```python
from build123d import *

# Parameters (mm, degrees)
SKETCH_1_W              = 40
SKETCH_1_H              = 40
EXTRUDE_1_DEPTH         = 20
SKETCH_2_R              = 6.58
EXTRUDE_2_DEPTH         = 1.8
SKETCH_3_R              = 2.925
EXTRUDE_3_DEPTH         = 3.8
SKETCH_4_W              = 7
SKETCH_4_H              = 20
EXTRUDE_4_DEPTH         = 2.4
HOLE_WIZARD_4_4_4_4_1_D = 4.4
SKETCH_7_W              = 5.7
SKETCH_7_H              = 4
EXTRUDE_5_DEPTH         = 8.5


with BuildPart() as part:
    # 草图1 → 凸台-拉伸1 (new body)
    with BuildSketch(Plane.XY):
        Rectangle(SKETCH_1_W, SKETCH_1_H)
    extrude(amount=EXTRUDE_1_DEPTH)

    # 草图2 → 凸台-拉伸2 (add)
    with BuildSketch(Plane(origin=(0, 20, 0), x_dir=(1, 0, 0), z_dir=(0, 1, 0))):
        with Locations((-10.3, -10)):
            Circle(SKETCH_2_R)
    extrude(amount=EXTRUDE_2_DEPTH)

    # 草图3 → 凸台-拉伸3 (add)
    with BuildSketch(Plane(origin=(0, 21.8, 0), x_dir=(1, 0, 0), z_dir=(0, 1, 0))):
        with Locations((-10.3, -10)):
            Circle(SKETCH_3_R)
    extrude(amount=EXTRUDE_3_DEPTH)

    # 草图4 → 凸台-拉伸4 (add)
    with BuildSketch(Plane(origin=(0, 12.2, 0), x_dir=(1, 0, 0), z_dir=(0, 1, 0))):
        with Locations((-23.5, -10)):
            Rectangle(SKETCH_4_W, SKETCH_4_H)
        with Locations((23.5, -10)):
            Rectangle(SKETCH_4_W, SKETCH_4_H)
    extrude(amount=-EXTRUDE_4_DEPTH)

    # Ø4.4 (4.4) 直径孔1 (through all)
    with Locations(Plane(origin=(0, 12.2, 0), x_dir=(1, 0, 0), z_dir=(0, 1, 0))):
        with Locations((-24.35, -4.95), (-24.35, -15.05), (24.35, -4.95), (24.35, -14.883974449)):
            Hole(HOLE_WIZARD_4_4_4_4_1_D / 2)

    # 草图7 → 凸台-拉伸5 (add)
    with BuildSketch(Plane.ZY.offset(20)):
        with Locations((10, -13.2)):
            Rectangle(SKETCH_7_W, SKETCH_7_H)
    extrude(amount=EXTRUDE_5_DEPTH)


solid = part.part
```
The listing builds one solid part. Answer for the finished solid, in the listing's coordinates (mm). A direction names the side the tool comes from. Coordinates: 2 decimals unless noted, no trailing zeros. Loops run counter-clockwise (first coordinate to the right, second up) from the corner with the lowest first, then second, coordinate; pieces in that order, holes last. Notation, with made-up numbers: (18, 36.5) -> (69, 36.5) arc R23 cw to (69, 64.5) -> close; hole circle Ø4 at (73.5, 25.5). An arc over 180 degrees is marked (long way). Return JSON: item names as keys, results as strings. Group by question number.
(1) A cutting plane is placed at A-A on x = -24.35. Write down the section's boundary in (y, z), and give its area (3 significant figures).
(2) Determine the mould class of faces 6 (the flat face through (0, 20, 10)), 7 (the cylindrical face through (-12.62, 23.67, 11.78)), 8 (the cylindrical face through (-25.37, 10.98, 17)), 9 (the cylindrical face through (-26.45, 10.98, 4.29)) for opening direction Z: released by +Z, released by -Z, zero draft, split by the parting line, or undercut.
(3) Given pin 1 Ø4 at (y, z) = (17, 7.5) entering from -X; pin 2 Ø2.5 at (y, z) = (15, 14.5) entering from +X; pin 3 Ø1.7 at (x, z) = (-22.5, 9) entering from -Y; pin 4 Ø2.5 at (x, z) = (24.35, 14.88) entering from +Y, each flat-ended and moving along its own axis, determine where each tip first touches the part or whether it passes through.
(4) A cutting plane is placed at B-B on z = 6.25. Write down the section's boundary in (x, y), and give its area (3 significant figures).
(5) Which of the six approach directions +Z, -Z, +X, -X, +Y, -Y give full straight-line access (tool end or side, diameter ignored) to faces 1 (the flat face through (-9, 21.8, 13)), 2 (the flat face through (-24, -11.2, 10)), 3 (the flat face through (-27, 11, 10)), 4 (the flat face through (-24, -13, 7.15)), 5 (the flat face through (23, 9.8, 10))?
(6) A cutting plane is placed at C-C on x = 24.35. Write down the section's boundary in (y, z), and give its area (3 significant figures).
(7) Find the intervals of material crossed by probe 1 along Z at (x, y) = (-24.35, 10.6); probe 2 along X at (y, z) = (11.3, 15.05); probe 3 along Y at (x, z) = (-24, 10.25), in increasing order. Write a range as from..to.
(8) A cutting plane is placed at D-D on z = 10. Write down the section's boundary in (x, y) (3 decimals).
The answers:
{
 "1": {"outline": "(-15.2, 7.15) -> (-11.2, 7.15) -> (-11.2, 12.85) -> (-15.2, 12.85) -> close; (9.8, 0) -> (12.2, 0) -> (12.2, 2.75) -> (9.8, 2.75) -> close; (9.8, 7.15) -> (12.2, 7.15) -> (12.2, 12.85) -> (9.8, 12.85) -> close; (9.8, 17.25) -> (12.2, 17.25) -> (12.2, 20) -> (9.8, 20) -> close", "area": "49.7 mm^2"},
 "2": {"face 6": "zero draft", "face 7": "split by the parting line", "face 8": "undercut", "face 9": "undercut"},
 "3": {"pin 1": "stops at x = -20", "pin 2": "stops at x = 20", "pin 3": "stops at y = -15.2", "pin 4": "passes through"},
 "4": {"outline": "(-27, 9.8) -> (-26.12, 9.8) -> (-26.12, 12.2) -> (-27, 12.2) -> close; (-22.58, 9.8) -> (-20, 9.8) -> (-20, -20) -> (20, -20) -> (20, 9.8) -> (22.58, 9.8) -> (22.58, 12.2) -> (20, 12.2) -> (20, 20) -> (-4.89, 20) -> (-4.89, 21.8) -> (-15.71, 21.8) -> (-15.71, 20) -> (-20, 20) -> (-20, 12.2) -> (-22.58, 12.2) -> close; (26.12, 9.8) -> (27, 9.8) -> (27, 12.2) -> (26.12, 12.2) -> close", "area": "1,640 mm^2"},
 "5": {"face 1": "+Y", "face 2": "+Z, -Z, -X", "face 3": "+Z, -Z, -X, +Y", "face 4": "-Z, -X, -Y", "face 5": "+Z, -Z, +X, -Y"},
 "6": {"outline": "(9.8, 0) -> (12.2, 0) -> (12.2, 2.75) -> (9.8, 2.75) -> close; (9.8, 7.15) -> (12.2, 7.15) -> (12.2, 12.68) -> (9.8, 12.68) -> close; (9.8, 17.08) -> (12.2, 17.08) -> (12.2, 20) -> (9.8, 20) -> close", "area": "26.9 mm^2"},
 "7": {"probe 1": "z = 0..2.75, 7.15..12.85, 17.25..20", "probe 2": "x = -27..-26.55, -22.15..22.16, 26.54..27", "probe 3": "y = -15.2..-11.2, 9.8..12.2"},
 "8": {"outline": "(-28.5, -15.2) -> (-20, -15.2) -> (-20, -20) -> (20, -20) -> (20, 9.8) -> (27, 9.8) -> (27, 12.2) -> (20, 12.2) -> (20, 20) -> (-3.72, 20) -> (-3.72, 21.8) -> (-7.375, 21.8) -> (-7.375, 25.6) -> (-13.225, 25.6) -> (-13.225, 21.8) -> (-16.88, 21.8) -> (-16.88, 20) -> (-20, 20) -> (-20, 12.2) -> (-27, 12.2) -> (-27, 9.8) -> (-20, 9.8) -> (-20, -11.2) -> (-28.5, -11.2) -> close"}
}
